The listing builds one solid part. Answer for the finished solid, in the listing's coordinates (mm). Face numbers are marked on the shaded views. A direction names the side the tool comes from. Round coordinates to 2 decimals unless told otherwise and drop trailing zeros. Write each loop counter-clockwise with the first axis right and the second up, starting at its lowest first coordinate (ties: lowest second). Pieces come first, ordered by that corner, then holes. Notation, with made-up numbers: (40.5, 51) - (58.5, 51) arc R18 ccw to (58.5, 70) - close; hole circle Ø2 at (-15, 15). An arc over 180 degrees is marked (long way). Return JSON: item names as keys, results as strings. Group by question number.
(1) Find the intervals of material crossed by line 1 along Y through (x, z) = (-11, -2.25); line 2 along X through (y, z) = (1, 4.5); line 3 along X through (y, z) = (-6.75, 1), in increasing order. Write a range as [from, to].
(2) Section D-D, the plane y = 26 is taken. Write down the section's boundary in (x, z), then the cut area to 3 significant figures.
(3) Determine the mould class of the marked faces 3, 4, 5 and 6 for opening direction X: +X half, -X half, draft (parallel to the pull), parting line (faces both ways), or undercut.
(4) Section B-B, the plane z = 1 is taken. Write down the section's boundary in (x, y).
(5) Which of the six approach directions +Z, -Z, +X, -X, +Y, -Y give full straight-line access (tool end or side, diameter ignored) to the marked faces 1 and 2?
(6) Each of these flat-tipped pins is pushed along its axis until it touches: pin 1 (4 mm diameter, centred on y = 5.5, z = 5, fed in from -X); pin 2 (6.5 mm diameter, centred on x = 1.5, y = 21.5, fed in from -Z); pin 3 (7.5 mm diameter, centred on x = -30, y = 1, fed in from +Z). Where does it stop, or does it pass through?
(7) Section C-C, the plane y = 38 is taken. Write down the section's boundary in (x, z), then the cut area to 3 significant figures.
(8) Section A-A, the plane x = 0 is taken. Write down the section's boundary in (y, z), then the cut area to 3 significant figures.
```python
from build123d import *

# Parameters (mm, degrees)
SKETCH1_W           = 100
SKETCH1_H           = 60
SKETCH1_R           = 4.25
SKETCH1_R_2         = 4
BOSS_EXTRUDE1_DEPTH = 7
SKETCH2_R           = 6.457332118
BOSS_EXTRUDE2_DEPTH = 6
CHAMFER1_SIZE       = 14
FILLET2_R           = 2.5
SKETCH3_W           = 30
SKETCH3_H           = 22
CUT_EXTRUDE1_DEPTH  = 6
SKETCH4_R           = 1.25
CUT_EXTRUDE2_DEPTH  = 12


with BuildPart() as part:
    # Sketch1 → Boss-Extrude1 (new body, symmetric)
    with BuildSketch(Plane.XY):
        with Locations((0, 20)):
            Rectangle(SKETCH1_W, SKETCH1_H)
        with Locations((30, 1)):
            Circle(SKETCH1_R, mode=Mode.SUBTRACT)
        with Locations((-30, 1)):
            Circle(SKETCH1_R, mode=Mode.SUBTRACT)
        with Locations((0, 39)):
            Circle(SKETCH1_R_2, mode=Mode.SUBTRACT)
    extrude(amount=BOSS_EXTRUDE1_DEPTH, both=True)

    # Sketch2 → Boss-Extrude2 (add)
    with BuildSketch(Plane(origin=(0, 0, -7), x_dir=(-1, 0, 0), z_dir=(0, 0, -1))):
        with Locations((-30, 1)):
            Circle(SKETCH2_R)
        with Locations((30, 1)):
            Circle(SKETCH2_R)
    extrude(amount=-BOSS_EXTRUDE2_DEPTH)

    # Chamfer1
    chamfer1_edges = [part.edges().sort_by_distance(p)[0] for p in [
        (50, -10, 0),
        (-50, -10, 0),
    ]]
    chamfer(chamfer1_edges, length=CHAMFER1_SIZE)

    # Fillet2
    fillet2_edges = [part.edges().sort_by_distance(p)[0] for p in [
        (0, -10, -7),
        (0, -10, 7),
        (-50, 27, 7),
        (50, 27, -7),
        (43, -3, -7),
        (-43, -3, -7),
        (50, 27, 7),
        (43, -3, 7),
        (-43, -3, 7),
        (-50, 27, -7),
    ]]
    fillet(fillet2_edges, radius=FILLET2_R)

    # Sketch3 → Cut-Extrude1 (cut)
    with BuildSketch(Plane(origin=(0, 0, -7), x_dir=(-1, 0, 0), z_dir=(0, 0, -1))):
        with Locations((0, 16.881077189)):
            Rectangle(SKETCH3_W, SKETCH3_H)
    extrude(amount=-CUT_EXTRUDE1_DEPTH, mode=Mode.SUBTRACT)

    # Sketch4 → Cut-Extrude2 (cut)
    with BuildSketch(Plane.XZ.offset(10)):
        with Locations((30, 1)):
            Circle(SKETCH4_R)
        with Locations((-30, 1)):
            Circle(SKETCH4_R)
    extrude(amount=-CUT_EXTRUDE2_DEPTH, mode=Mode.SUBTRACT)


solid = part.part
```
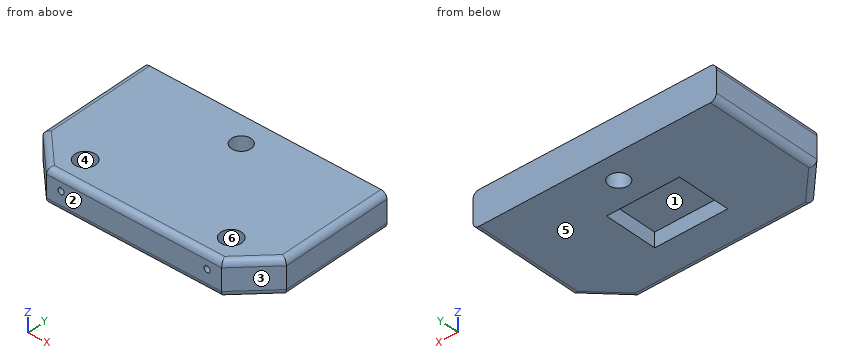
Working result:
{
 "1": {"line 1": "y = [-10, 5.88], [27.88, 50]", "line 2": "x = [-47, -34.25], [-25.75, 25.75], [34.25, 47]", "line 3": "x = [-39.25, -31.25], [-28.75, 28.75], [31.25, 39.25]"},
 "2": {"outline": "(-50, -4.5) arc R2.5 ccw to (-47.5, -7) - (-15, -7) - (-15, -1) - (15, -1) - (15, -7) - (47.5, -7) arc R2.5 ccw to (50, -4.5) - (50, 4.5) arc R2.5 ccw to (47.5, 7) - (-47.5, 7) arc R2.5 ccw to (-50, 4.5) - close", "area": "1,210 mm^2"},
 "3": {"face 3": "+X half", "face 4": "undercut", "face 5": "draft", "face 6": "undercut"},
 "4": {"outline": "(-50, 4) - (-36, -10) - (-31.25, -10) - (-31.25, -3.06) arc R4.25 cw (long way) to (-28.75, -3.06) - (-28.75, -10) - (28.75, -10) - (28.75, -3.06) arc R4.25 cw (long way) to (31.25, -3.06) - (31.25, -10) - (36, -10) - (50, 4) - (50, 50) - (-50, 50) - close; hole circle Ø8 at (0, 39)"},
 "5": {"face 1": "-Z", "face 2": "+Z, -Z, +X, -X, -Y"},
 "6": {"pin 1": "stops at x = -50", "pin 2": "stops at z = -1", "pin 3": "stops at z = -1"},
 "7": {"outline": "(-50, -4.5) arc R2.5 ccw to (-47.5, -7) - (-3.87, -7) - (-3.87, 7) - (-47.5, 7) arc R2.5 ccw to (-50, 4.5) - close; (3.87, -7) - (47.5, -7) arc R2.5 ccw to (50, -4.5) - (50, 4.5) arc R2.5 ccw to (47.5, 7) - (3.87, 7) - close", "area": "1,290 mm^2"},
 "8": {"outline": "(-10, -4.5) arc R2.5 ccw to (-7.5, -7) - (5.88, -7) - (5.88, -1) - (27.88, -1) - (27.88, -7) - (35, -7) - (35, 7) - (-7.5, 7) arc R2.5 ccw to (-10, 4.5) - close; (43, -7) - (50, -7) - (50, 7) - (43, 7) - close", "area": "593 mm^2"}
}
